The listing builds one solid part. Answer for the finished solid, in the listing's coordinates (mm). Face numbers are marked on the shaded views. A direction names the side the tool comes from. Round coordinates to 2 decimals unless told otherwise and drop trailing zeros. Write each loop counter-clockwise with the first axis right and the second up, starting at its lowest first coordinate (ties: lowest second). Pieces come first, ordered by that corner, then holes. Notation, with made-up numbers: (-5, 16) - (52, 16) arc R24 ccw to (52, 34) - close; hole circle Ø3 at (70, 65.5). An arc over 180 degrees is marked (long way). Use a Markdown table: item, result. Add a question column.
1) A cutting plane is placed at A-A (y = 10.4). Give the vertices of the cut face in (x, z).
2) A cutting plane is placed at C-C (z = -7.5). Give the vertices of the cut face in (x, y), then the cut area to 3 significant figures.
3) A cutting plane is placed at D-D (z = -1.25). Give the vertices of the cut face in (x, y), then the cut area to 3 significant figures.
4) Each of these flat-tipped pins is pushed along its axis until it touches: P1, Ø5, axis at x = 17.9, z = -7.5, coming from the +Y side; P2, Ø2.5, axis at y = 17.9, z = -7.5, coming from the +X side. Where does it stop, or does it pass through?
5) Find the intervals of material crossed by probe 1 along X at (y, z) = (0.9, -7.5); probe 2 along Y at (x, z) = (16.75, -1.5), in increasing order. Write a range as from..to.
6) A tool of negligible diameter and unlimited length cuts with its end or side. For the marked faces 1 and 2, from which of +Z, -Z, +X, -X, +Y, -Y can it reach the whole face along a straight path? Write none if from no direction.
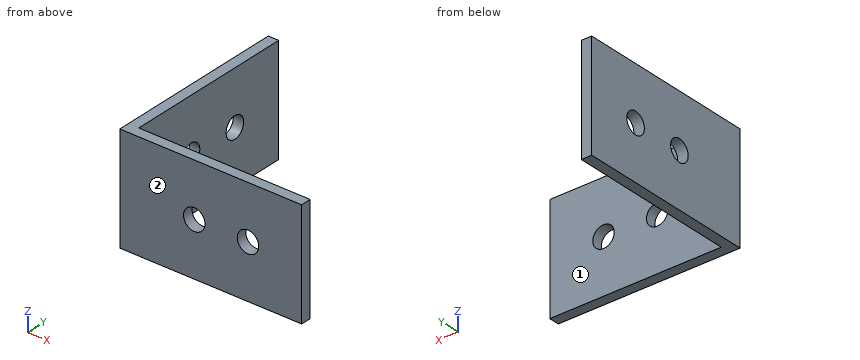
```python
from build123d import *

# Parameters (mm, degrees)
SKETCH1_W           = 15
SKETCH1_H           = 25.4
BOSS_EXTRUDE1_DEPTH = 3.175
SKETCH2_W           = 15
SKETCH2_H           = 3.175
BOSS_EXTRUDE2_DEPTH = 22.225
SKETCH4_R           = 1.5
CUT_EXTRUDE3_DEPTH  = 37.933868265
SKETCH3_R           = 1.5
CUT_EXTRUDE4_DEPTH  = 39.927111375
SKETCH7_W           = 22.225
SKETCH7_H           = 15
CUT_EXTRUDE7_DEPTH  = 1.7145
SKETCH8_W           = 15
SKETCH8_H           = 23.9395
CUT_EXTRUDE8_DEPTH  = 1.7145


with BuildPart() as part:
    # Sketch1 → Boss-Extrude1 (new body)
    with BuildSketch(Plane(origin=(0, 0, 0), x_dir=(0, 0, -1), z_dir=(1, 0, 0))):
        with Locations((7.5, 12.7)):
            Rectangle(SKETCH1_W, SKETCH1_H)
    extrude(amount=BOSS_EXTRUDE1_DEPTH)

    # Sketch2 → Boss-Extrude2 (add)
    with BuildSketch(Plane(origin=(3.175, 0, 0), x_dir=(0, 0, -1), z_dir=(1, 0, 0))):
        with Locations((7.5, 1.5875)):
            Rectangle(SKETCH2_W, SKETCH2_H)
    extrude(amount=BOSS_EXTRUDE2_DEPTH)

    # Sketch4 → Cut-Extrude3 (cut, through all)
    with BuildSketch(Plane(origin=(3.175, 0, 0), x_dir=(0, 0, -1), z_dir=(1, 0, 0))):
        with Locations((7.5, 17.9)):
            Circle(SKETCH4_R)
        with Locations((7.5, 10.4)):
            Circle(SKETCH4_R)
    extrude(amount=-CUT_EXTRUDE3_DEPTH, mode=Mode.SUBTRACT)

    # Sketch3 → Cut-Extrude4 (cut, through all)
    with BuildSketch(Plane.XZ):
        with Locations(Location((10.4, -7.5, 0), (0, 0, 270))):
            Circle(SKETCH3_R)
        with Locations(Location((17.9, -7.5, 0), (0, 0, 270))):
            Circle(SKETCH3_R)
    extrude(amount=-CUT_EXTRUDE4_DEPTH, mode=Mode.SUBTRACT)

    # Sketch7 → Cut-Extrude7 (cut)
    with BuildSketch(Plane(origin=(0, 3.175, 0), x_dir=(1, 0, 0), z_dir=(0, 1, 0))):
        with Locations((14.2875, 7.5)):
            Rectangle(SKETCH7_W, SKETCH7_H)
    extrude(amount=-CUT_EXTRUDE7_DEPTH, mode=Mode.SUBTRACT)

    # Sketch8 → Cut-Extrude8 (cut)
    with BuildSketch(Plane(origin=(3.175, 0, 0), x_dir=(0, 0, -1), z_dir=(1, 0, 0))):
        with Locations((7.5, 13.43025)):
            Rectangle(SKETCH8_W, SKETCH8_H)
    extrude(amount=-CUT_EXTRUDE8_DEPTH, mode=Mode.SUBTRACT)


solid = part.part
```
Entries:
| question | item | result |
|---|---|---|
| 1 | outline | (0, -15) - (1.46, -15) - (1.46, -9) - (0, -9) - close; (0, -6) - (1.46, -6) - (1.46, 0) - (0, 0) - close |
| 2 | outline | (0, 0) - (8.9, 0) - (8.9, 1.46) - (1.46, 1.46) - (1.46, 8.9) - (0, 8.9) - close; (0, 11.9) - (1.46, 11.9) - (1.46, 16.4) - (0, 16.4) - close; (0, 19.4) - (1.46, 19.4) - (1.46, 25.4) - (0, 25.4) - close; (11.9, 0) - (16.4, 0) - (16.4, 1.46) - (11.9, 1.46) - close; (19.4, 0) - (25.4, 0) - (25.4, 1.46) - (19.4, 1.46) - close |
| 2 | area | 54.5 mm² |
| 3 | outline | (0, 0) - (25.4, 0) - (25.4, 1.46) - (1.46, 1.46) - (1.46, 25.4) - (0, 25.4) - close |
| 3 | area | 72.1 mm² |
| 4 | P1 | stops at y = 1.46 |
| 4 | P2 | passes through |
| 5 | probe 1 | x = 0..8.9, 11.9..16.4, 19.4..25.4 |
| 5 | probe 2 | y = 0..1.46 |
| 6 | face 1 | +Z, -Z, +X, +Y |
| 6 | face 2 | +Z, -Z, +X, -X, -Y |
